from build123d import *

# Parameters (mm, degrees)
CROQUIS1_W              = 12
CROQUIS1_H              = 20
CROQUIS1_W_2            = 26
CROQUIS1_H_2            = 16
SALIENTE_EXTRUIR1_DEPTH = 2
CROQUIS2_W              = 27
CROQUIS2_H              = 25
SALIENTE_EXTRUIR2_DEPTH = 14.6
CROQUIS3_W              = 27
CROQUIS3_H              = 13.6
CORTAR_EXTRUIR1_DEPTH   = 2
REDONDEO1_R             = 3
REDONDEO2_R             = 2
CROQUIS4_W              = 8
CROQUIS4_H              = 12.6
CORTAR_EXTRUIR2_DEPTH   = 2
CROQUIS5_W              = 8
CROQUIS5_H              = 12.6
CORTAR_EXTRUIR3_DEPTH   = 2
CROQUIS6_R              = 0.75
CORTAR_EXTRUIR4_DEPTH   = 2
CROQUIS7_R              = 0.9
SALIENTE_EXTRUIR3_DEPTH = 16.6
CROQUIS8_R              = 0.9
CORTAR_EXTRUIR5_DEPTH   = 6


with BuildPart() as part:
    # Croquis1 → Saliente-Extruir1 (new body)
    with BuildSketch(Plane(origin=(0, 0, 0), x_dir=(1, 0, 0), z_dir=(0, 1, 0))):
        Polygon((31, 29), (31, -30), (0, -30), (0, 0), (-46, 0), (-46, 29), align=None)
        with Locations((-33, 14.5)):
            Rectangle(CROQUIS1_W, CROQUIS1_H, mode=Mode.SUBTRACT)
        with Locations((-11, 14.5)):
            Rectangle(CROQUIS1_W_2, CROQUIS1_H_2, mode=Mode.SUBTRACT)
    extrude(amount=SALIENTE_EXTRUIR1_DEPTH)

    # Croquis2 → Saliente-Extruir2 (add)
    with BuildSketch(Plane(origin=(0, 2, 0), x_dir=(1, 0, 0), z_dir=(0, 1, 0))):
        Polygon((0, -30), (31, -30), (31, 29), (-46, 29), (-46, 24), (-44, 24), (-44, 27), (23.5, 27), (23.5, 2), (-44, 2), (-44, 5), (-46, 5), (-46, 0), (0, 0), align=None)
        with Locations((15.5, -15.5)):
            Rectangle(CROQUIS2_W, CROQUIS2_H, mode=Mode.SUBTRACT)
    extrude(amount=SALIENTE_EXTRUIR2_DEPTH)

    # Croquis3 → Cortar-Extruir1 (cut)
    with BuildSketch(Plane.XY.offset(30)):
        with Locations((15.5, 9.8)):
            Rectangle(CROQUIS3_W, CROQUIS3_H)
    extrude(amount=-CORTAR_EXTRUIR1_DEPTH, mode=Mode.SUBTRACT)

    # Redondeo1
    redondeo1_edges = [part.edges().sort_by_distance(p)[0] for p in [
        (0, 8.3, 0),
        (-46, 8.3, 0),
        (-46, 8.3, -29),
        (31, 8.3, -29),
    ]]
    fillet(redondeo1_edges, radius=REDONDEO1_R)

    # Redondeo2
    redondeo2_edges = [part.edges().sort_by_distance(p)[0] for p in [
        (-44, 9.3, -27),
        (23.5, 9.3, -27),
        (23.5, 9.3, -2),
        (-44, 9.3, -2),
        (29, 9.3, 3),
        (2, 9.3, 3),
    ]]
    fillet(redondeo2_edges, radius=REDONDEO2_R)

    # Croquis4 → Cortar-Extruir2 (cut)
    with BuildSketch(Plane.XY):
        with Locations((-34, 10.3)):
            Rectangle(CROQUIS4_W, CROQUIS4_H)
    extrude(amount=-CORTAR_EXTRUIR2_DEPTH, mode=Mode.SUBTRACT)

    # Croquis5 → Cortar-Extruir3 (cut)
    with BuildSketch(Plane(origin=(0, 0, -29), x_dir=(-1, 0, 0), z_dir=(0, 0, -1))):
        with Locations((11, 10.3)):
            Rectangle(CROQUIS5_W, CROQUIS5_H)
    extrude(amount=-CORTAR_EXTRUIR3_DEPTH, mode=Mode.SUBTRACT)

    # Croquis6 → Cortar-Extruir4 (cut)
    with BuildSketch(Plane(origin=(0, 2, 0), x_dir=(1, 0, 0), z_dir=(0, 1, 0))):
        with Locations(Location((26, -6, 0), (0, 0, 270))):
            Circle(CROQUIS6_R)
        with Locations(Location((5, -6, 0), (0, 0, 270))):
            Circle(CROQUIS6_R)
        with Locations(Location((5, -19.2, 0), (0, 0, 270))):
            Circle(CROQUIS6_R)
        with Locations(Location((26, -19.2, 0), (0, 0, 270))):
            Circle(CROQUIS6_R)
    extrude(amount=-CORTAR_EXTRUIR4_DEPTH, mode=Mode.SUBTRACT)

    # Croquis7 → Saliente-Extruir3 (add)
    # profile 1 of 4: a face of its own
    with BuildSketch(Plane(origin=(0, 16.6, 0), x_dir=(1, 0, 0), z_dir=(0, 1, 0))):
        with BuildLine():
            Line((31, -30), (31, -24))
            ThreePointArc((31, -24), (31.292893219, -24.707106781), (32, -25))
            ThreePointArc((32, -25), (34.5, -27.5), (32, -30))
            Line((32, -30), (31, -30))
        make_face()
        with Locations(Location((32, -27.5, 0), (0, 0, 270))):
            Circle(CROQUIS7_R, mode=Mode.SUBTRACT)
    # profile 2 of 4: a face of its own
    with BuildSketch(Plane(origin=(0, 16.6, 0), x_dir=(1, 0, 0), z_dir=(0, 1, 0))):
        with BuildLine():
            Line((-1, -30), (0, -30))
            Line((0, -30), (0, -24))
            ThreePointArc((0, -24), (-0.292893219, -24.707106781), (-1, -25))
            ThreePointArc((-1, -25), (-3.5, -27.5), (-1, -30))
        make_face()
        with Locations(Location((-1, -27.5, 0), (0, 0, 90))):
            Circle(CROQUIS7_R, mode=Mode.SUBTRACT)
    # profile 3 of 4: a face of its own
    with BuildSketch(Plane(origin=(0, 16.6, 0), x_dir=(1, 0, 0), z_dir=(0, 1, 0))):
        with BuildLine():
            Line((-34.5, 29), (-41.5, 29))
            ThreePointArc((-41.5, 29), (-40.792893219, 29.292893219), (-40.5, 30))
            ThreePointArc((-40.5, 30), (-38, 32.5), (-35.5, 30))
            ThreePointArc((-35.5, 30), (-35.207106781, 29.292893219), (-34.5, 29))
        make_face()
        with Locations(Location((-38, 30, 0), (0, 0, 270))):
            Circle(CROQUIS7_R, mode=Mode.SUBTRACT)
    # profile 4 of 4: a face of its own
    with BuildSketch(Plane(origin=(0, 16.6, 0), x_dir=(1, 0, 0), z_dir=(0, 1, 0))):
        with BuildLine():
            Line((-21.5, 0), (-28.5, 0))
            ThreePointArc((-28.5, 0), (-27.792893219, -0.292893219), (-27.5, -1))
            ThreePointArc((-27.5, -1), (-25, -3.5), (-22.5, -1))
            ThreePointArc((-22.5, -1), (-22.207106781, -0.292893219), (-21.5, 0))
        make_face()
        with Locations(Location((-25, -1, 0), (0, 0, 90))):
            Circle(CROQUIS7_R, mode=Mode.SUBTRACT)
    extrude(amount=-SALIENTE_EXTRUIR3_DEPTH)

    # Croquis8 → Cortar-Extruir5 (cut)
    with BuildSketch(Plane(origin=(0, 16.6, 0), x_dir=(1, 0, 0), z_dir=(0, 1, 0))):
        with Locations(Location((28, 26, 0), (0, 0, 270))):
            Circle(CROQUIS8_R)
    extrude(amount=-CORTAR_EXTRUIR5_DEPTH, mode=Mode.SUBTRACT)


solid = part.part
CAD build for the part. Positions are in the model's coordinates, mm. A direction names the side the tool comes from. Give positions to 0.01 mm unless a question says otherwise; leave off trailing zeros. Order: outer loops, then holes, each group sorted by start corner. A loop starts at its lowest first (then second) coordinate and runs counter-clockwise, first axis right, second up. Notation, with made-up numbers: (17.5, 88.5) - (32.5, 88.5) arc R19 cw to (32.5, 94.5) - close; hole circle Ø7 at (-26.75, -17.5). An arc over 180 degrees is marked (long way). Write each question's results on one line, items separated by ' | '.
1. Pin check, flat tips, straight feed: pin 1 (1.6 mm diameter, centred on x = -12.5, z = -28.5, fed in from +Y); pin 2 (1 mm diameter, centred on y = 1, z = -11.5, fed in from +X); pin 3 (7.5 mm diameter, centred on y = 13, z = 18, fed in from -X). Stop position of each tip, or through.
Calculated:
pin 1: stops at y = 4 | pin 2: stops at x = 31 | pin 3: stops at x = 0
2. Saw through at B-B on x = -25. List the corners of the cut face in (y, z), and give its area (3 significant figures).
Calculated:
outline: (0, -29) - (16.6, -29) - (16.6, -27) - (2, -27) - (2, -2) - (16.6, -2) - (16.6, 0.1) - (0, 0.1) - close; (0, 1.9) - (16.6, 1.9) - (16.6, 3.5) - (0, 3.5) - close | area: 145 mm2
3. Saw through at A-A on z = -16. List the corners of the cut face in (x, y), and give its area (4 significant figures).
Calculated:
outline: (-46, 0) - (-39, 0) - (-39, 2) - (-46, 2) - close; (-27, 0) - (-24, 0) - (-24, 2) - (-27, 2) - close; (2, 0) - (31, 0) - (31, 16.6) - (23.5, 16.6) - (23.5, 2) - (2, 2) - close | area: 187.5 mm2
4. Saw through at D-D on x = 18. List the corners of the cut face in (y, z).
Calculated:
outline: (0, -29) - (16.6, -29) - (16.6, -27) - (2, -27) - (2, -2) - (16.6, -2) - (16.6, 3) - (2, 3) - (2, 28) - (3, 28) - (3, 30) - (0, 30) - close
5. Saw through at C-C on y = 7.5. Count the separate pieces of the cut face and the enclosed holes in it, and give its area (3 significant figures).
Calculated:
separate pieces: 3 | enclosed holes: 4 | area: 728 mm2
6. Probe L1, parallel to X at y = 11.75, z = 27.5; L2, parallel to Z at x = -25, y = 11.25; L3, parallel to X at y = 0.65, z = 6. List the from-to ranges inside material, lowest first. Write a range as from..to.
Calculated:
L1: x = -3.5..-1.9, -0.1..2, 29..31.1, 32.9..34.5 | L2: z = -29..-27, -2..0.1, 1.9..3.5 | L3: x = 0..4.25, 5.75..25.25, 26.75..31
7. 3-axis set-ups, long thin cutter, end or side, ignore diameter. For faces 1 (the face through (-15, 10, -28)), 2 (the face through (-33, 1, -24.5)), 3 (the face through (-11, 3, -27)), 4 (the face through (-30, 10, -1)), 5 (the face through (-45, 9, -24)): which of +Z, -Z, +X, -X, +Y, -Y reach the whole face in a straight line?
Calculated:
face 1: -Z, +Y | face 2: +Y, -Y | face 3: +Y | face 4: +Z, +Y | face 5: -X, +Y
8. Pull direction X, two halves, no side cores. Call faces 6 (the face through (34.5, 8.4, 27.4)), 7 (the face through (-24, 1, -14)), 8 (the face through (29, 9, 18)), 9 (the face through (12, 16.6, -1.8)): released by +X, released by -X, zero draft, split by the parting line, or undercut.
Calculated:
face 6: released by +X | face 7: undercut | face 8: undercut | face 9: zero draft
